The listing builds one solid part. Answer for the finished solid, in the listing's coordinates (mm). A direction names the side the tool comes from. Give positions to 0.01 mm unless a question says otherwise; leave off trailing zeros. Loops run counter-clockwise (first coordinate to the right, second up) from the corner with the lowest first, then second, coordinate; pieces in that order, holes last. Notation, with made-up numbers: (83, -8) - (131, -8) arc R25 cw to (131, 14) - close; hole circle Ø5 at (80, 69). An arc over 180 degrees is marked (long way). Write item = value, one per line. Start each with the question number.
1) The part is cut by section C-C on y = 4. State how many separate pieces and enclosed holes the cut face has, plus the area to 3 significant figures.
2) The mould has two halves that part along X. Classify faces 4 (the cylindrical face through (-44.504, 3.451, -1.709)), 5 (the flat face through (-35, 4, -0.6)), 6 (the flat face through (-3, 3, -13.5)): +X half, -X half, draft (parallel to the pull), parting line (faces both ways), or undercut.
3) Which of the six approach directions +Z, -Z, +X, -X, +Y, -Y give full straight-line access (tool end or side, diameter ignored) to faces 1 (the flat face through (-10.6, 5, 7.7)), 2 (the cylindrical face through (-7.81, 5.42, -1.73)), 3 (the flat face through (-30.613, 4, 4))?
4) Flat-ended cylindrical pins translate along their axes: P1, Ø5, axis at x = 25, z = 2.5, coming from the -Y side; P2, Ø3, axis at x = -16, z = 22, coming from the +Y side; P3, Ø1.6, axis at x = 12.5, y = 6.5, coming from the +Z side. Find the tip coordinate at first contact, or state that the pin passes through.
5) The part is cut by section B-B on x = -12. Write down the section's boundary in (y, z).
6) The part is cut by section D-D on x = -27. Write down the section's boundary in (y, z).
7) Consider probe 1 along X at (y, z) = (12.7, 0); probe 2 along X at (y, z) = (2.25, 9); probe 3 along X at (y, z) = (1.85, 9). Determine where each line is inside the solid, lowest interval first.
from build123d import *

# Parameters (mm, degrees)
SKETCH3_R               = 8
SKETCH3_W               = 54.803
SKETCH3_H               = 32
SKETCH3_R_2             = 5
BOSS_EXTRUDE1_DEPTH     = 7
CUT_EXTRUDE3_DEPTH      = 65.105926161
CUT_EXTRUDE3_DEPTH_BACK = 65.105926161
SKETCH4_R               = 1.75
SKETCH6_R               = 11
SKETCH6_R_2             = 8
BOSS_EXTRUDE2_DEPTH     = 4
SKETCH7_R               = 11
SKETCH7_R_2             = 5
BOSS_EXTRUDE3_DEPTH     = 3
CHAMFER1_SIZE           = 2.5
CUT_EXTRUDE5_DEPTH      = 66.242392422
CUT_EXTRUDE5_DEPTH_BACK = 66.242392422
SKETCH9_R               = 1.75
CUT_EXTRUDE6_START      = -2
SKETCH10_R              = 1.75
CUT_EXTRUDE6_DEPTH      = 2
CHAMFER3_SIZE2          = 32
CHAMFER3_SIZE           = 22
CHAMFER4_SIZE           = 16
FILLET1_DEPTH           = 7
BOSS_EXTRUDE6_START     = -5
SKETCH15_R              = 10.5
BOSS_EXTRUDE6_DEPTH     = 5


with BuildPart() as part:
    # Sketch3 → Boss-Extrude1 (new body)
    # profile 1 of 10: a face of its own
    with BuildSketch(Plane(origin=(0, 0, 0), x_dir=(1, 0, 0), z_dir=(0, 1, 0))):
        with BuildLine():
            ThreePointArc((-17.613, 0), (-21.567058454, 9.545941546), (-31.113, 13.5))
            Line((-31.113, 13.5), (-31.113, 10.5))
            ThreePointArc((-31.113, 10.5), (-23.688378798, 7.424621202), (-20.613, 0))
            ThreePointArc((-20.613, 0), (-23.688378798, -7.424621202), (-31.113, -10.5))
            Line((-31.113, -10.5), (-31.113, -13.5))
            ThreePointArc((-31.113, -13.5), (-21.567058454, -9.545941546), (-17.613, 0))
        make_face()
    # profile 2 of 10: a face of its own
    with BuildSketch(Plane(origin=(0, 0, 0), x_dir=(1, 0, 0), z_dir=(0, 1, 0))):
        with BuildLine():
            Line((-31.113, 10.5), (-31.113, 13.5))
            ThreePointArc((-31.113, 13.5), (-44.613, 0), (-31.113, -13.5))
            Line((-31.113, -13.5), (-31.113, -10.5))
            ThreePointArc((-31.113, -10.5), (-41.613, 0), (-31.113, 10.5))
        make_face()
    # profile 3 of 10: a face of its own
    with BuildSketch(Plane(origin=(0, 0, 0), x_dir=(1, 0, 0), z_dir=(0, 1, 0))):
        with BuildLine():
            Line((23.69, 13.5), (-31.113, 13.5))
            ThreePointArc((-31.113, 13.5), (-21.567058454, 9.545941546), (-17.613, 0))
            ThreePointArc((-17.613, 0), (-21.567058454, -9.545941546), (-31.113, -13.5))
            Line((-31.113, -13.5), (23.69, -13.5))
            Line((23.69, -13.5), (23.69, -11))
            ThreePointArc((23.69, -11), (12.69, 0), (23.69, 11))
            Line((23.69, 11), (23.69, 13.5))
        make_face()
        with Locations(Location((0, 0, 0), (0, 0, 270))):
            Circle(SKETCH3_R, mode=Mode.SUBTRACT)
    # profile 4 of 10: a face of its own
    with BuildSketch(Plane(origin=(0, 0, 0), x_dir=(1, 0, 0), z_dir=(0, 1, 0))):
        with BuildLine():
            ThreePointArc((-17.613, 0), (-21.567058454, 9.545941546), (-31.113, 13.5))
            Line((-31.113, 13.5), (-31.113, 10.5))
            ThreePointArc((-31.113, 10.5), (-23.688378798, 7.424621202), (-20.613, 0))
            ThreePointArc((-20.613, 0), (-23.688378798, -7.424621202), (-31.113, -10.5))
            Line((-31.113, -10.5), (-31.113, -13.5))
            ThreePointArc((-31.113, -13.5), (-21.567058454, -9.545941546), (-17.613, 0))
        make_face()
    # profile 5 of 10: a face of its own
    with BuildSketch(Plane(origin=(0, 0, 0), x_dir=(1, 0, 0), z_dir=(0, 1, 0))):
        with BuildLine():
            Line((-31.113, 10.5), (-31.113, 13.5))
            ThreePointArc((-31.113, 13.5), (-44.613, 0), (-31.113, -13.5))
            Line((-31.113, -13.5), (-31.113, -10.5))
            ThreePointArc((-31.113, -10.5), (-41.613, 0), (-31.113, 10.5))
        make_face()
    # profile 6 of 10: a face of its own
    with BuildSketch(Plane(origin=(0, 0, 0), x_dir=(1, 0, 0), z_dir=(0, 1, 0))):
        with BuildLine():
            ThreePointArc((34.69, 0), (31.468174593, 7.778174593), (23.69, 11))
            Line((23.69, 11), (23.69, 8))
            ThreePointArc((23.69, 8), (29.346854249, 5.656854249), (31.69, 0))
            ThreePointArc((31.69, 0), (29.346854249, -5.656854249), (23.69, -8))
            Line((23.69, -8), (23.69, -11))
            ThreePointArc((23.69, -11), (31.468174593, -7.778174593), (34.69, 0))
        make_face()
    # profile 7 of 10: a face of its own
    with BuildSketch(Plane(origin=(0, 0, 0), x_dir=(1, 0, 0), z_dir=(0, 1, 0))):
        with BuildLine():
            Line((23.69, 8), (23.69, 11))
            ThreePointArc((23.69, 11), (12.69, 0), (23.69, -11))
            Line((23.69, -11), (23.69, -8))
            ThreePointArc((23.69, -8), (15.69, 0), (23.69, 8))
        make_face()
    # profile 8 of 10: a face of its own
    with BuildSketch(Plane(origin=(0, 0, 0), x_dir=(1, 0, 0), z_dir=(0, 1, 0))):
        with Locations((-3.7115, -29.5)):
            Rectangle(SKETCH3_W, SKETCH3_H)
        with Locations(Location((0, -32.707574931, 0), (0, 0, 270))):
            Circle(SKETCH3_R_2, mode=Mode.SUBTRACT)
    # profile 9 of 10: a face of its own
    with BuildSketch(Plane(origin=(0, 0, 0), x_dir=(1, 0, 0), z_dir=(0, 1, 0))):
        with BuildLine():
            ThreePointArc((34.69, 0), (31.468174593, 7.778174593), (23.69, 11))
            Line((23.69, 11), (23.69, 8))
            ThreePointArc((23.69, 8), (29.346854249, 5.656854249), (31.69, 0))
            ThreePointArc((31.69, 0), (29.346854249, -5.656854249), (23.69, -8))
            Line((23.69, -8), (23.69, -11))
            ThreePointArc((23.69, -11), (31.468174593, -7.778174593), (34.69, 0))
        make_face()
    # profile 10 of 10: a face of its own
    with BuildSketch(Plane(origin=(0, 0, 0), x_dir=(1, 0, 0), z_dir=(0, 1, 0))):
        with BuildLine():
            Line((23.69, 8), (23.69, 11))
            ThreePointArc((23.69, 11), (12.69, 0), (23.69, -11))
            Line((23.69, -11), (23.69, -8))
            ThreePointArc((23.69, -8), (15.69, 0), (23.69, 8))
        make_face()
    extrude(amount=BOSS_EXTRUDE1_DEPTH)

    # Sketch4 → Cut-Extrude3 (cut, two sides: drawn at the far end of the back side and taken through both)
    with BuildSketch(Plane(origin=(0, 0, 0), x_dir=(1, 0, 0), z_dir=(0, 1, 0)).offset(-CUT_EXTRUDE3_DEPTH_BACK)):
        with Locations(Location((5.5, -27.207574931, 0), (0, 0, 270))):
            Circle(SKETCH4_R)
        with Locations(Location((5.5, -38.207574931, 0), (0, 0, 270))):
            Circle(SKETCH4_R)
        with Locations(Location((-5.5, -38.207574931, 0), (0, 0, 270))):
            Circle(SKETCH4_R)
        with Locations(Location((-5.5, -27.207574931, 0), (0, 0, 270))):
            Circle(SKETCH4_R)
    extrude(amount=CUT_EXTRUDE3_DEPTH + CUT_EXTRUDE3_DEPTH_BACK, mode=Mode.SUBTRACT)

    # Sketch6 → Boss-Extrude2 (add)
    # profile 1 of 2: a face of its own
    with BuildSketch(Plane(origin=(0, 7, 0), x_dir=(1, 0, 0), z_dir=(0, 1, 0))):
        with Locations(Location((23.69, 0, 0), (0, 0, 270))):
            Circle(SKETCH6_R)
        with Locations(Location((23.69, 0, 0), (0, 0, 270))):
            Circle(SKETCH6_R_2, mode=Mode.SUBTRACT)
    # profile 2 of 2: a face of its own
    with BuildSketch(Plane(origin=(0, 7, 0), x_dir=(1, 0, 0), z_dir=(0, 1, 0))):
        with Locations(Location((0, 0, 0), (0, 0, 270))):
            Circle(SKETCH6_R)
        with Locations(Location((0, 0, 0), (0, 0, 270))):
            Circle(SKETCH6_R_2, mode=Mode.SUBTRACT)
    extrude(amount=BOSS_EXTRUDE2_DEPTH)

    # Sketch7 → Boss-Extrude3 (add)
    # profile 1 of 2: a face of its own
    with BuildSketch(Plane(origin=(0, 11, 0), x_dir=(1, 0, 0), z_dir=(0, 1, 0))):
        with Locations(Location((23.69, 0, 0), (0, 0, 270))):
            Circle(SKETCH7_R)
        with Locations(Location((23.69, 0, 0), (0, 0, 270))):
            Circle(SKETCH7_R_2, mode=Mode.SUBTRACT)
    # profile 2 of 2: a face of its own
    with BuildSketch(Plane(origin=(0, 11, 0), x_dir=(1, 0, 0), z_dir=(0, 1, 0))):
        with Locations(Location((0, 0, 0), (0, 0, 270))):
            Circle(SKETCH7_R)
        with Locations(Location((0, 0, 0), (0, 0, 270))):
            Circle(SKETCH7_R_2, mode=Mode.SUBTRACT)
    extrude(amount=BOSS_EXTRUDE3_DEPTH)

    # Chamfer1
    # the kernel refuses this chamfer: 2.5 mm, written as the material it adds along each edge
    with BuildSketch(Plane(origin=(23.69, 0, -11), x_dir=(0.9912092295509807, 0, 0.13230367815352426), z_dir=(0, 1, 0))) as chamfer1_piece_1_section:
        with BuildLine():
            Line((2.910680919, 0), (-CHAMFER1_SIZE * 0.132303678154, CHAMFER1_SIZE * 0.991209229551))
            Line((-CHAMFER1_SIZE * 0.132303678154, CHAMFER1_SIZE * 0.991209229551), (0, 0))
            ThreePointArc((0, 0), (1.49552658, 0.096625069), (2.910680919, 0))
        make_face()
    chamfer1_piece_1 = extrude(amount=7, mode=Mode.PRIVATE)
    chamfer1_piece_1 = split(chamfer1_piece_1, bisect_by=Plane(origin=(23.69, 0, -13.5), z_dir=(0, 0, 1)), keep=Keep.TOP, mode=Mode.PRIVATE)
    add(chamfer1_piece_1)

    # Sketch9 → Cut-Extrude5 (cut, two sides: drawn at the far end of the back side and taken through both)
    with BuildSketch(Plane(origin=(0, 0, 0), x_dir=(1, 0, 0), z_dir=(0, 1, 0)).offset(-CUT_EXTRUDE5_DEPTH_BACK)):
        with Locations(Location((12, 9, 0), (0, 0, 90))):
            Circle(SKETCH9_R)
        with Locations(Location((12, -9, 0), (0, 0, 90))):
            Circle(SKETCH9_R)
        with Locations(Location((-12, -9, 0), (0, 0, 90))):
            Circle(SKETCH9_R)
        with Locations(Location((-12, 9, 0), (0, 0, 90))):
            Circle(SKETCH9_R)
    extrude(amount=CUT_EXTRUDE5_DEPTH + CUT_EXTRUDE5_DEPTH_BACK, mode=Mode.SUBTRACT)

    # Sketch10 → Cut-Extrude6 (cut)
    # profile 1 of 4: a face of its own
    with BuildSketch(Plane(origin=(0, 7, 0), x_dir=(1, 0, 0), z_dir=(0, 1, 0)).offset(CUT_EXTRUDE6_START)):
        Polygon((-15.175426481, -9), (-13.58771324, -11.75), (-10.41228676, -11.75), (-8.824573519, -9), (-10.41228676, -6.25), (-13.58771324, -6.25), align=None)
        with Locations(Location((-12, -9, 0), (0, 0, 90))):
            Circle(SKETCH10_R, mode=Mode.SUBTRACT)
    # profile 2 of 4: a face of its own
    with BuildSketch(Plane(origin=(0, 7, 0), x_dir=(1, 0, 0), z_dir=(0, 1, 0)).offset(CUT_EXTRUDE6_START)):
        Polygon((-15.175426481, 9), (-13.58771324, 6.25), (-10.41228676, 6.25), (-8.824573519, 9), (-10.41228676, 11.75), (-13.58771324, 11.75), align=None)
        with Locations(Location((-12, 9, 0), (0, 0, 90))):
            Circle(SKETCH10_R, mode=Mode.SUBTRACT)
    # profile 3 of 4: a face of its own
    with BuildSketch(Plane(origin=(0, 7, 0), x_dir=(1, 0, 0), z_dir=(0, 1, 0)).offset(CUT_EXTRUDE6_START)):
        Polygon((15.175426481, 9), (13.58771324, 11.75), (10.41228676, 11.75), (8.824573519, 9), (10.41228676, 6.25), (13.58771324, 6.25), align=None)
        with Locations(Location((12, 9, 0), (0, 0, 90))):
            Circle(SKETCH10_R, mode=Mode.SUBTRACT)
    # profile 4 of 4: a face of its own
    with BuildSketch(Plane(origin=(0, 7, 0), x_dir=(1, 0, 0), z_dir=(0, 1, 0)).offset(CUT_EXTRUDE6_START)):
        Polygon((15.175426481, -9), (13.58771324, -6.25), (10.41228676, -6.25), (8.824573519, -9), (10.41228676, -11.75), (13.58771324, -11.75), align=None)
        with Locations(Location((12, -9, 0), (0, 0, 90))):
            Circle(SKETCH10_R, mode=Mode.SUBTRACT)
    extrude(amount=CUT_EXTRUDE6_DEPTH, mode=Mode.SUBTRACT)

    # Chamfer2
    # the kernel refuses this chamfer: 5 mm, written as the material it adds along each edge
    with BuildSketch(Plane(origin=(23.69, 0, 11), x_dir=(0.9874000606639179, 0, -0.15824386307497393), z_dir=(0, 1, 0))) as chamfer2_piece_1:
        with BuildLine():
            Line((3.622786344, 0.141421356), (-0.805837357, -4.287202344))
            Line((-0.805837357, -4.287202344), (-0.904577363, -4.271377958))
            ThreePointArc((-0.904577363, -4.271377958), (-0.443767224, -2.137054655), (-0.098740006, 0.015824386))
            Line((-0.098740006, 0.015824386), (0.015824386, 0.098740006))
            ThreePointArc((0.015824386, 0.098740006), (1.81210794, -0.038365312), (3.606961958, 0.240161362))
            Line((3.606961958, 0.240161362), (3.622786344, 0.141421356))
        make_face()
    extrude(amount=7)

    # Chamfer3
    chamfer3_edges = [part.edges().sort_by_distance(p)[0] for p in [
        (-31.113, 3.5, 45.5),
    ]]
    chamfer3_side = [part.faces().sort_by_distance(p)[0] for p in [
        (-30.673, 3.5, 45.5),
    ]]
    chamfer(chamfer3_edges, length=CHAMFER3_SIZE - 0.0001, length2=CHAMFER3_SIZE2 - 0.0001, reference=chamfer3_side[0])  # a hair under: the kernel refuses the full size

    # Chamfer4
    chamfer4_edges = [part.edges().sort_by_distance(p)[0] for p in [
        (23.69, 3.5, 45.5),
    ]]
    chamfer(chamfer4_edges, length=CHAMFER4_SIZE)

    # Fillet1: read off the stored shape, not the designer's step
    # Fillet1 outline → Fillet1 (add)
    with BuildSketch(Plane(origin=(0, 0, 0), x_dir=(1, 0, 0), z_dir=(0, 1, 0))):
        with BuildLine():
            ThreePointArc((-31.113, -13.5), (-32.547033058, -13.423619079), (-33.96483904, -13.19534062))
            ThreePointArc((-33.96483904, -13.19534062), (-31.199410591, -14.370304214), (-29.062482337, -16.482571146))
            Line((-29.062482337, -16.482571146), (-31.113, -13.5))
        make_face()
    extrude(amount=FILLET1_DEPTH)

    # Sketch15 → Boss-Extrude6 (add)
    with BuildSketch(Plane(origin=(0, 7, 0), x_dir=(1, 0, 0), z_dir=(0, 1, 0)).offset(BOSS_EXTRUDE6_START)):
        with Locations(Location((-31.113, 0, 0), (0, 0, 270))):
            Circle(SKETCH15_R)
        Polygon((-31.613, 0.6), (-31.613, 8), (-30.613, 8), (-30.613, 0.6), (-23.113, 0.6), (-23.113, -0.6), (-30.613, -0.6), (-30.613, -8), (-31.613, -8), (-31.613, -0.6), (-39.113, -0.6), (-39.113, 0.6), align=None, mode=Mode.SUBTRACT)
    extrude(amount=BOSS_EXTRUDE6_DEPTH)


solid = part.part
Answer below:
q1.separate_pieces = 1
q1.enclosed_holes = 12
q1.area = 2,650 mm2
q2.face_4 = -X half
q2.face_5 = undercut
q2.face_6 = draft
q3.face_1 = +Y
q3.face_2 = -Y
q3.face_3 = +Y, -Y
q4.P1 = 11
q4.P2 = 7
q4.P3 = 41.49
q5.outline = (0, -13.5) - (7, -13.5) - (7, -11.75) - (5, -11.75) - (5, -10.75) - (0, -10.75) - close; (0, -7.25) - (5, -7.25) - (5, -6.25) - (7, -6.25) - (7, 6.25) - (5, 6.25) - (5, 7.25) - (0, 7.25) - close; (0, 10.75) - (5, 10.75) - (5, 11.75) - (7, 11.75) - (7, 41.3) - (0, 41.3) - close
q6.outline = (0, -13.5) - (7, -13.5) - (7, -0.6) - (2, -0.6) - (2, -9.66) - (0, -9.66) - close; (0, 9.66) - (2, 9.66) - (2, 0.6) - (7, 0.6) - (7, 19.48) - (0, 19.48) - close
q7.probe_1 = -11 to -5, 5 to 11, 12.69 to 18.69, 28.69 to 34.69
q7.probe_2 = -41.18 to -13.75, -10.25 to 10.25, 13.75 to 30.01
q7.probe_3 = -41.18 to -36.52, -25.7 to -13.75, -10.25 to 10.25, 13.75 to 30.01
